from build123d import *

# Parameters (mm, degrees)
F0_W     = 317
F0_H     = 585
F1_DEPTH = 334
F2_W     = 115
F2_H     = 110
F3_DEPTH = 15
F4_W     = 115
F4_H     = 110
F5_DEPTH = 15


with BuildPart() as f1:
    # F0 (on Front) → F1 (new body, symmetric)
    with BuildSketch(Plane.XZ):
        with Locations((158.5, 292.5)):
            Rectangle(F0_W, F0_H)
    extrude(amount=F1_DEPTH, both=True)

    # F2 (on face) → F3 (join)
    with BuildSketch(Plane.XZ.offset(334)):
        with Locations((158.5, 475)):
            Rectangle(F2_W, F2_H)
        with Locations((158.5, 145)):
            Rectangle(F2_W, F2_H)
    extrude(amount=F3_DEPTH)

    # F4 (on face) → F5 (join)
    with BuildSketch(Plane(origin=(0, 334, 0), x_dir=(-1, 0, 0), z_dir=(0, 1, 0))):
        with Locations((-158.5, 475)):
            Rectangle(F4_W, F4_H)
        with Locations((-158.5, 145)):
            Rectangle(F4_W, F4_H)
    extrude(amount=F5_DEPTH)


solid = f1.part
Geometry: final body of the model. Coordinates: model frame, mm. A direction names the side the tool comes from. Round coordinates to 2 decimals unless told otherwise and drop trailing zeros. Write each loop counter-clockwise with the first axis right and the second up, starting at its lowest first coordinate (ties: lowest second). Pieces come first, ordered by that corner, then holes. Notation, with made-up numbers: M 24.25,52 L 66.25,52 A17 cw 66.25,76 Z; hole C 15.25,78.25 d11. An arc over 180 degrees is marked long. Write item = value, one per line.
Item 1: Access query for faces 5 (the face through (216, -341, 474)), 6 (the face through (158, -341, 530)), 7 (the face through (158, -341, 420)). Directions: +Z, -Z, +X, -X, +Y, -Y. A direction counts if a zero-diameter tool reaches every point of the face in a straight line with its end or side. Return the directions, or none.
Findings:
face_5 = +Z, -Z, +X, -Y
face_6 = +Z, +X, -X, -Y
face_7 = +X, -X, -Y
Item 2: Section query A-A on x = 208. Return loops of the section in (y, z).
Findings:
outline = M -349,90 L -334,90 L -334,0 L 334,0 L 334,90 L 349,90 L 349,200 L 334,200 L 334,420 L 349,420 L 349,530 L 334,530 L 334,585 L -334,585 L -334,530 L -349,530 L -349,420 L -334,420 L -334,200 L -349,200 Z
Item 3: Pin query (flat end, axial travel): P1, Ø16.5, axis at y = 343, z = 119, coming from the +X side; P2, Ø12, axis at y = 341.5, z = 136.5, coming from the -X side; P3, Ø7.5, axis at x = 186.5, y = 338, coming from the +Z side. Return the tip coordinate at first contact, or that it passes through.
Findings:
P1 = 216
P2 = 101
P3 = 530
Item 4: Material intervals for line 1 along Y through (x, z) = (235, 29.5), sorted ascending. Write a range as [from, to].
Findings:
line_1 = [-334, 334]
Item 5: Section query C-C on z = 65. Return loops of the section in (x, y), then the cut area to 3 significant figures.
Findings:
outline = M 0,-334 L 317,-334 L 317,334 L 0,334 Z
area = 212,000 mm^2
Item 6: Pull-direction query (Z, two-part tool) for faces 1 (the face through (156, -5, 0)), 2 (the face through (216, -341, 144)), 3 (the face through (156, 334, 297)), 4 (the face through (158, -341, 200)); classes: pulls with the +Z half, pulls with the -Z half, needs draft (parallel to the pull), parting line crosses it, or undercut.
Findings:
face_1 = pulls with the -Z half
face_2 = needs draft
face_3 = undercut
face_4 = undercut
Item 7: Section query B-B on z = 448.5. Return loops of the section in (x, y).
Findings:
outline = M 0,-334 L 101,-334 L 101,-349 L 216,-349 L 216,-334 L 317,-334 L 317,334 L 216,334 L 216,349 L 101,349 L 101,334 L 0,334 Z
Item 8: Section query D-D on x = 264.5. Return loops of the section in (y, z).
Findings:
outline = M -334,0 L 334,0 L 334,585 L -334,585 Z
